Geometry check sheet. Reference: the model listing, model coordinates, mm. Coordinates: 2 decimals unless noted, no trailing zeros. Loops run counter-clockwise (first coordinate to the right, second up) from the corner with the lowest first, then second, coordinate; pieces in that order, holes last.
from build123d import *

# Parameters (mm, degrees)
SKETCH1_W           = 78
SKETCH1_H           = 49
BOSS_EXTRUDE1_DEPTH = 1.6
SKETCH2_R           = 8.951195902
CUT_EXTRUDE1_DEPTH  = 10
SKETCH4_W           = 1.6
SKETCH4_H           = 31.097608196
BOSS_EXTRUDE3_DEPTH = 2
SKETCH5_R           = 0.968115871
SKETCH5_R_2         = 1.048792193
SKETCH5_R_3         = 0.324209478
SKETCH5_R_4         = 0.640689511
SKETCH5_R_5         = 0.655195162
SKETCH5_R_6         = 0.453768234
SKETCH5_R_7         = 0.5
SKETCH5_R_8         = 0.4826
SKETCH5_R_9         = 0.635
CUT_EXTRUDE2_DEPTH  = 10
SKETCH6_R           = 2
CUT_EXTRUDE3_DEPTH  = 10


with BuildPart() as part:
    # Sketch1 → Boss-Extrude1 (new body)
    with BuildSketch(Plane.XY):
        Rectangle(SKETCH1_W, SKETCH1_H)
    extrude(amount=BOSS_EXTRUDE1_DEPTH)

    # Sketch2 → Cut-Extrude1 (cut)
    with BuildSketch(Plane.XY.offset(1.6)):
        with Locations((39, 24.5)):
            Circle(SKETCH2_R)
        with Locations((39, -24.5)):
            Circle(SKETCH2_R)
        with Locations((-39, 24.5)):
            Circle(SKETCH2_R)
        with Locations((-39, -24.5)):
            Circle(SKETCH2_R)
    extrude(amount=-CUT_EXTRUDE1_DEPTH, mode=Mode.SUBTRACT)

    # Sketch4 → Boss-Extrude3 (add)
    with BuildSketch(Plane(origin=(39, 0, 0), x_dir=(0, 0, -1), z_dir=(1, 0, 0))):
        with Locations((-0.8, 0)):
            Rectangle(SKETCH4_W, SKETCH4_H)
    extrude(amount=BOSS_EXTRUDE3_DEPTH)

    # Sketch5 → Cut-Extrude2 (cut)
    with BuildSketch(Plane(origin=(0, 0, 0), x_dir=(-1, 0, 0), z_dir=(0, 0, -1))):
        with Locations((-22.850936129, 20.463344351)):
            Circle(SKETCH5_R)
        with Locations((-11.32352045, 20.463344351)):
            Circle(SKETCH5_R_2)
        with Locations((-20.469685942, 14.979253011)):
            Circle(SKETCH5_R_3)
        with Locations((26.963692039, -3.596337313)):
            Circle(SKETCH5_R_4)
        with Locations((26.963692039, 3.820462687)):
            Circle(SKETCH5_R_5)
        with Locations((33.083891647, 8.744582154)):
            Circle(SKETCH5_R_6)
        with Locations((33.083891647, 13.778350388)):
            Circle(SKETCH5_R_7)
        with Locations((23.383432149, -9.480592582)):
            Circle(SKETCH5_R_8)
        with Locations((23.383432149, -6.940592582)):
            Circle(SKETCH5_R_8)
        with Locations((-39.570851538, 3.081777689)):
            Circle(SKETCH5_R_7)
        with Locations((-37.030851538, 0.541777689)):
            Circle(SKETCH5_R_9)
    extrude(amount=-CUT_EXTRUDE2_DEPTH, mode=Mode.SUBTRACT)

    # Sketch6 → Cut-Extrude3 (cut)
    with BuildSketch(Plane.XY.offset(1.6)):
        with Locations((25.232939878, -15.376639124)):
            Circle(SKETCH6_R)
        with Locations((-25.028046678, -15.376639124)):
            Circle(SKETCH6_R)
        with Locations((-25.028046678, 15.720969071)):
            Circle(SKETCH6_R)
        with Locations((25.232939878, 15.720969071)):
            Circle(SKETCH6_R)
    extrude(amount=-CUT_EXTRUDE3_DEPTH, mode=Mode.SUBTRACT)


solid = part.part
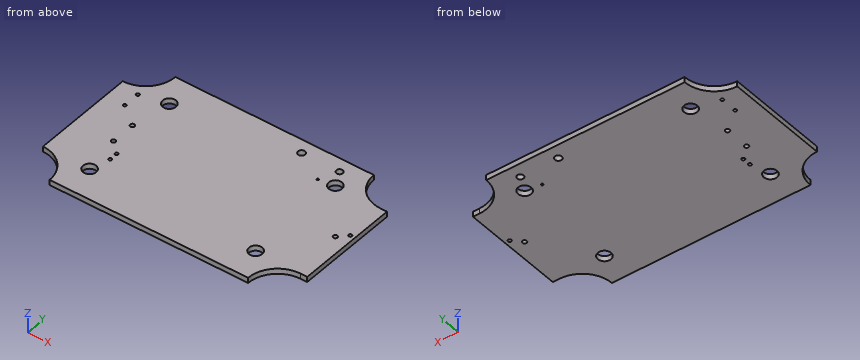
(1) Sectioned sample at B-B on z = 0.75. State how many separate pieces and enclosed holes the cut face has, and give its area (3 significant figures).
Findings:
separate pieces: 1
enclosed holes: 15
area: 3,570 mm2
(2) Gauge pin test, flat end, axial feed: pin 1 Ø2 at (x, y) = (22.85, 20.46) entering from +Z. Record the tip position at first contact, or that the pin passes through.
Findings:
pin 1: stops at z = 1.6
(3) Sectioned sample at A-A on y = -16.5. Record the cut outline in (x, z), and give its area (3 significant figures).
Findings:
outline: (-34.98, 0) - (-26.68, 0) - (-26.68, 1.6) - (-34.98, 1.6) - close; (-23.37, 0) - (23.58, 0) - (23.58, 1.6) - (-23.37, 1.6) - close; (26.89, 0) - (34.98, 0) - (34.98, 1.6) - (26.89, 1.6) - close
area: 101 mm2
(4) Scan lines: L1, parallel to Y at x = -24, z = 0.95; L2, parallel to X at y = -15, z = 0.6; L3, parallel to Y at x = 26, z = 0.95. Record each from-to range of solid material in increasing order.
Findings:
L1: y = -24.5 to -17.09, -13.66 to 14.01, 17.44 to 24.5
L2: x = -39 to -26.99, -23.06 to 23.27, 27.2 to 41
L3: y = -24.5 to -17.22, -13.53 to 13.87, 17.57 to 24.5
